Check sheet for the modelled part. Datum: model origin and axes. Units: mm. A direction names the side the tool comes from. Round coordinates to 2 decimals unless told otherwise and drop trailing zeros. Order: outer loops, then holes, each group sorted by start corner. A loop starts at its lowest first (then second) coordinate and runs counter-clockwise, first axis right, second up. Notation, with made-up numbers: (-23.75, -13.75) -> (-17.75, -13.75) arc R23 ccw to (-17.75, 8.25) -> close; hole circle Ø7 at (-23.5, -20). An arc over 180 degrees is marked (long way). Answer in a Markdown table with one row per item.
```python
from build123d import *

# Parameters (mm, degrees)
SKETCH1_R             = 87.5
BOSS_EXTRUDE1_DEPTH   = 29
SKETCH2_R             = 15
CUT_EXTRUDE1_DEPTH    = 128.096420091
SKETCH3_R             = 7.666988893
CUT_EXTRUDE2_DEPTH    = 21.221625
CIRPATTERN1_START     = 7.778375175
CIRPATTERN1_OUTLINE_R = 7.666988893
CIRPATTERN1_DEPTH     = 21.221624825


# Read off the part's stored shape, not the designer's step: CirPattern1
with BuildPart() as part:
    # Sketch1 → Boss-Extrude1 (new body)
    with BuildSketch(Plane(origin=(0, 0, 0), x_dir=(1, 0, 0), z_dir=(0, 1, 0))):
        with Locations(Location((0, 0, 0), (0, 0, 90))):
            Circle(SKETCH1_R)
    extrude(amount=BOSS_EXTRUDE1_DEPTH)

    # Sketch2 → Cut-Extrude1 (cut, through all)
    with BuildSketch(Plane(origin=(0, 0, 0), x_dir=(1, 0, 0), z_dir=(0, 1, 0))):
        with Locations(Location((0, 0, 0), (0, 0, 90))):
            Circle(SKETCH2_R)
    extrude(amount=CUT_EXTRUDE1_DEPTH, mode=Mode.SUBTRACT)

    # Sketch3 → Cut-Extrude2 (cut)
    with BuildSketch(Plane(origin=(0, 29, 0), x_dir=(1, 0, 0), z_dir=(0, 1, 0))):
        with Locations(Location((-35.094392614, 0, 0), (0, 0, 270))):
            Circle(SKETCH3_R)
    extrude(amount=-CUT_EXTRUDE2_DEPTH, mode=Mode.SUBTRACT)

    # CirPattern1 outline → CirPattern1 (cut)
    with BuildSketch(Plane(origin=(0, 0, 0), x_dir=(1, 0, 0), z_dir=(0, 1, 0)).offset(CIRPATTERN1_START)):
        with Locations((17.547196307, 30.392635534)):
            Circle(CIRPATTERN1_OUTLINE_R)
        with Locations((17.547196307, -30.392635534)):
            Circle(CIRPATTERN1_OUTLINE_R)
    extrude(amount=CIRPATTERN1_DEPTH, mode=Mode.SUBTRACT)


solid = part.part
```
(1) Depth check by flat-ended pin: pin 1 Ø24.5 at (x, z) = (17.55, 30.39) entering from -Y; pin 2 Ø7.5 at (x, z) = (16.5, 33) entering from +Y; pin 3 Ø6 at (x, y) = (13, 25.5) entering from +Z; pin 4 Ø4 at (y, z) = (22.5, -69) entering from -X. Enter the tip coordinate at first touch or a pass-through.
Solutions:
| item | result |
|---|---|
| pin 1 | y = 0 |
| pin 2 | y = 7.78 |
| pin 3 | z = 86.93 |
| pin 4 | x = -56.28 |
(2) Section check C-C on y = 24.25. Record the boundary of the cut face in (x, z), plus the area to 3 significant figures.
Solutions:
| item | result |
|---|---|
| outline | circle Ø175 at (0, 0); hole circle Ø15.33 at (-35.09, 0); hole circle Ø30 at (0, 0); hole circle Ø15.33 at (17.55, -30.39); hole circle Ø15.33 at (17.55, 30.39) |
| area | 22,800 mm^2 |
(3) Section check A-A on x = 0. Record the boundary of the cut face in (y, z).
Solutions:
| item | result |
|---|---|
| outline | (0, -87.5) -> (29, -87.5) -> (29, -15) -> (0, -15) -> close; (0, 15) -> (29, 15) -> (29, 87.5) -> (0, 87.5) -> close |
(4) Draft check along X on faces 3 (the cylindrical face through (-86.755, 14.297, 11.391)), 4 (the cylindrical face through (-0.66, 14.297, 14.985)), 5 (the flat face through (18, 29, 1)). Enter one of: pulls with the +X half, pulls with the -X half, needs draft (parallel to the pull), parting line crosses it, or undercut.
Solutions:
| item | result |
|---|---|
| face 3 | parting line crosses it |
| face 4 | undercut |
| face 5 | needs draft |
(5) Tool access check on faces 1 (the flat face through (17, 7.778, 30)), 2 (the flat face through (-1, 0, -18)). Record the directions out of +Z, -Z, +X, -X, +Y, -Y that give a thin tool (end or side, any length) a straight path to the whole face; none if there is none.
Solutions:
| item | result |
|---|---|
| face 1 | +Y |
| face 2 | +Z, -Z, +X, -X, -Y |
(6) Section check D-D on z = 36. Record the boundary of the cut face in (x, y).
Solutions:
| item | result |
|---|---|
| outline | (-79.75, 0) -> (79.75, 0) -> (79.75, 29) -> (22.78, 29) -> (22.78, 7.78) -> (12.32, 7.78) -> (12.32, 29) -> (-79.75, 29) -> close |
(7) Section check B-B on z = 0. Record the boundary of the cut face in (x, y), plus the area to 3 significant figures.
Solutions:
| item | result |
|---|---|
| outline | (-87.5, 0) -> (-15, 0) -> (-15, 29) -> (-27.43, 29) -> (-27.43, 7.78) -> (-42.76, 7.78) -> (-42.76, 29) -> (-87.5, 29) -> close; (15, 0) -> (87.5, 0) -> (87.5, 29) -> (15, 29) -> close |
| area | 3,880 mm^2 |
(8) Scan lines: probe 1 along X at (y, z) = (15.5, 0); probe 2 along Z at (x, y) = (-37, 9); probe 3 along Z at (x, y) = (-7, 3.75). Record each from-to range of solid material in increasing order. Write a range as from..to.
Solutions:
| item | result |
|---|---|
| probe 1 | -87.5..-42.76, -27.43..-15, 15..87.5 |
| probe 2 | -79.29..-7.43, 7.43..79.29 |
| probe 3 | -87.22..-13.27, 13.27..87.22 |
